Autodesk Inventor part; units mm, degrees
ref_plane "YZ Plane" through (0, 0, 0) normal (1, 0, 0) x (0, 1, 0)
ref_plane "XZ Plane" through (0, 0, 0) normal (0, 1, 0) x (-1, 0, 0)
ref_plane "XY Plane" through (0, 0, 0) normal (0, 0, 1) x (1, 0, 0)
sketch "Sketch1" plane through (0, 0, 0) normal (0, 0, 1) x (1, 0, 0)
  line L0 (-18.2895, 105.4386) -> (-13.2895, 105.4386)
  line L1 (-13.2895, 105.4386) -> (-13.2895, 5.4386)
  line L2 (-18.2895, 84.1228) -> (-18.2895, 105.4386)
  line L3 (-13.2895, 5.4386) -> (26.7105, 5.4386)
  line L4 (26.7105, 5.4386) -> (26.7105, 0.4386)
  line L5 (26.7105, 0.4386) -> (-18.2895, 0.4386)
  line L6 (-18.2895, 0.4386) -> (-18.2895, 84.1228)
  point P0 (0, 0)
  dimension "d0" = 5
  dimension "d1" = 5
  dimension "d2" = 100
  dimension "d3" = 40
extrude "Extrusion1" add sketch "Sketch1" along normal blind 30
fillet "Fillet1" radius 4 2 edges at (-18.2895, 0.4386, 15) (-13.2895, 5.4386, 15)
sketch "Sketch2" plane through (-13.2895, 105.4386, 30) normal (1, 0, 0) x (0, 0, -1)
  circle A0 centre (15, -10) radius 3.1
  line L0 (30, -96) -> (30, 0)
  line L1 (30, 0) -> (0, 0)
  circle A1 centre (15, -25) radius 3.1
  circle A2 centre (15, -40) radius 3.1
  circle A3 centre (15, -55) radius 3.1
  circle A4 centre (15, -70) radius 3.1
  point P0 (30, -105.4386)
  dimension "d7" = 6.2
  dimension "d8" = 15
  dimension "d9" = 10
  dimension "d13" = 15
extrude "Extrusion2" cut sketch "Sketch2" against normal through all
sketch "Sketch3" plane through (26.7105, 5.4386, 30) normal (0, 1, 0) x (1, 0, 0)
  arc A0 (-29.9118, 10.4403) -> (-25.9203, 5.7011) centre (-28, 8) ccw
  arc A1 (-10.0083, 19.2121) -> (-13.3603, 24.3717) centre (-11.364, 22) ccw
  line L0 (-25.9203, 5.7011) -> (-8.8328, 20.2103)
  line L1 (-30.0783, 10.3002) -> (-13.3603, 24.3717)
  line L2 (0, 30) -> (-36, 30)
  line L3 (0, 0) -> (-36, 0)
  line L4 (0, 30) -> (0, 0)
  line L5 (-36, 0) -> (-36, 30)
  point P0 (-26.7105, 30)
  dimension "d20" = 6.2
  dimension "d21" = 6.2
  dimension "d22" = 8
  dimension "d23" = 8
  dimension "d24" = 11.364
  dimension "d25" = 8
extrude "Extrusion3" cut sketch "Sketch3" against normal through all contours L1 A1 L0 A0
properties part number "Mounting Bracket"
For this review, take the finished solid that the model builds, in its own axes (mm). A direction names the side the tool comes from. Round coordinates to 2 decimals unless told otherwise and drop trailing zeros. Write each loop counter-clockwise with the first axis right and the second up, starting at its lowest first coordinate (ties: lowest second). Pieces come first, ordered by that corner, then holes. Notation, with made-up numbers: (7, -6.5) - (54, -6.5) arc R15 ccw to (54, -1.5) - close; hole circle Ø4 at (-39.75, -1.5). An arc over 180 degrees is marked (long way). Use CSV: the item, a comma, the result in double quotes.
1) Add section D-D on y = 27. Write out the cut boundary in (x, z), and give its area (3 significant figures).
Conclusion:
outline,"(-18.29, 0) - (-13.29, 0) - (-13.29, 30) - (-18.29, 30) - close"
area,"150 mm^2"
2) For faces 4 (the flat face through (26.71, 3, 15)), 5 (the flat face through (4.96, 2.97, 12.69)), 6 (the flat face through (-13.29, 58, 15)), list the 3-axis set-ups (+Z, -Z, +X, -X, +Y, -Y) from which the entire face can be reached by the end or side of a thin tool; tool diameter is ignored.
Conclusion:
face 4,"+Z, -Z, +X, +Y, -Y"
face 5,"+Y, -Y"
face 6,"+Z, -Z, +X, +Y"
3) Add section C-C on z = 3.5. Write out the cut boundary in (x, y).
Conclusion:
outline,"(-18.29, 4.44) arc R4 ccw to (-14.29, 0.44) - (26.71, 0.44) - (26.71, 5.44) - (-9.29, 5.44) arc R4 cw to (-13.29, 9.44) - (-13.29, 105.44) - (-18.29, 105.44) - close"
4) The part is to be moulded in two halves that separate along Z. For faces 1 (the flat face through (-14, 42, 0)), 2 (the cylindrical face through (-15.754, 68.512, 15.404)), 3 (the flat face through (1.9, 0.439, 14.8)), say which applies: pulls with the +Z half, pulls with the -Z half, needs draft (parallel to the pull), parting line crosses it, or undercut.
Conclusion:
face 1,"pulls with the -Z half"
face 2,"undercut"
face 3,"needs draft"
5) Wall thickness on line 1 along Y through (x, z) = (-16.4, 15); line 2 along Y through (x, z) = (-16.6, 15); line 3 along Y through (x, z) = (17.5, 12.5): over which ranges is each line inside the solid? List them lowest first. Write a range as from..to.
Conclusion:
line 1,"y = 1.04..32.34, 38.54..47.34, 53.54..62.34, 68.54..77.34, 83.54..92.34, 98.54..105.44"
line 2,"y = 1.17..32.34, 38.54..47.34, 53.54..62.34, 68.54..77.34, 83.54..92.34, 98.54..105.44"
line 3,"y = 0.44..5.44"
6) Clearance check with flat-ended pins moving along their axes: pin 1 Ø8 at (y, z) = (50.44, 15) entering from +X; pin 2 Ø4 at (x, z) = (11.5, 5.5) entering from +Y. State where each tip first meets the part, or that it passes through.
Conclusion:
pin 1,"stops at x = -13.29"
pin 2,"stops at y = 5.44"
7) Add section B-B on z = 15. Count the separate pieces of the cut face and the enclosed holes in it, and give its area (3 significant figures).
Conclusion:
separate pieces,"7"
enclosed holes,"0"
area,"522 mm^2"
8) Add section A-A on z = 7.75. Write out the cut boundary in (x, y).
Conclusion:
outline,"(-18.29, 4.44) arc R4 ccw to (-14.29, 0.44) - (10.83, 0.44) - (10.83, 5.44) - (-9.29, 5.44) arc R4 cw to (-13.29, 9.44) - (-13.29, 105.44) - (-18.29, 105.44) - close; (18.44, 0.44) - (26.71, 0.44) - (26.71, 5.44) - (18.44, 5.44) - close"
